Autodesk Fusion 360 part; units mm, degrees
sketch "Sketch1" plane through (0, 0, 0) normal (0, 0, 1) x (1, 0, 0)
  line L0 (-25, 35) -> (19, 35)
  line L1 (19, 35) -> (19, -79)
  line L2 (19, -79) -> (-25, -79)
  line L3 (-25, -79) -> (-25, 35)
  line L4 (-25, 35) -> (-32.5, 35)
  line L5 (-32.5, 35) -> (-32.5, 42.5)
  line L6 (-32.5, 42.5) -> (-25, 42.5)
  line L7 (-25, 42.5) -> (-25, 35)
  line L8 (-32.5, 42.5) -> (26.5, 42.5)
  line L9 (26.5, 42.5) -> (26.5, -86.5)
  line L10 (26.5, -86.5) -> (-32.5, -86.5)
  line L11 (-32.5, -86.5) -> (-32.5, 42.5)
  dimension "d1" = 44
  dimension "d2" = 114
  dimension "d3" = 7.5
  dimension "d4" = 7.5
  dimension "d5" = 59
  dimension "d6" = 129
extrude "Extrude1" add sketch "Sketch1" along normal blind 7 contours L0 L1 L2 L3 | L4 L7 L8 L9 L10 L11 | L4 L5 L6 L7 L8 L11 makes body 1
sketch "Sketch2" plane through (0, 0, 0) normal (0, 0, 1) x (1, 0, 0)
  circle A0 centre (-25, -79) radius 7
  circle A1 centre (19, -79) radius 7
  circle A2 centre (19, 35) radius 7
  circle A3 centre (-25, 35) radius 7
  point P0 (-25, -79)
  point P1 (19, -79)
  point P2 (19, 35)
  point P3 (-25, 35)
  dimension "d9" = 14
  dimension "d10" = 14
  dimension "d11" = 14
  dimension "d12" = 14
extrude "Extrude2" cut sketch "Sketch2" along normal blind 4 contours A0 bodies 1
extrude "Extrude3" cut sketch "Sketch2" along normal blind 4 contours A1 bodies 1
extrude "Extrude4" cut sketch "Sketch2" along normal blind 4 contours A3 bodies 1
extrude "Extrude5" cut sketch "Sketch2" along normal blind 4 contours A2 bodies 1
sketch "Sketch3" plane through (0, 0, 0) normal (0, 0, 1) x (1, 0, 0)
hole "Hole1" at (-25, -79, 4) direction (0, 0, 1) diameter 4 depth 10 tip angle 118 bodies 1
hole "Hole2" at (19, -79, 4) direction (0, 0, 1) diameter 4 depth 10 tip angle 118 bodies 1
hole "Hole3" at (19, 35, 4) direction (0, 0, 1) diameter 4 depth 10 tip angle 118 bodies 1
hole "Hole4" at (-25, 35, 4) direction (0, 0, 1) diameter 4 depth 10 tip angle 118 bodies 1
extrude "Extrude6" add 1 faces at (-12.8333, 42.5, 2.3333) along direction (0, 1, 0) blind 10.5 on bodies 1 bodies 1
extrude "Extrude7" add 1 faces at (6.8333, -86.5, 2.3333) along direction (0, -1, 0) blind 10.5 on bodies 1 bodies 1
sketch "Sketch4" plane through (0, 0, 0) normal (0, 0, -1) x (1, 0, 0)
  circle A0 centre (19, -35) radius 7
  circle A1 centre (-25, -35) radius 7
  circle A2 centre (19, 79) radius 7
  circle A3 centre (-25, 79) radius 7
  line L0 (-32.5, 97) -> (-32.5, -53)
  line L1 (-32.5, -53) -> (26.5, -53)
  line L2 (26.5, -53) -> (26.5, 97)
  line L3 (26.5, 97) -> (-32.5, 97)
  line L4 (-32.5, -53) -> (26.5, -53)
  line L5 (26.5, -53) -> (26.5, 17)
  line L6 (26.5, 17) -> (-32.5, 17)
  line L7 (-32.5, 17) -> (-32.5, -53)
  line L8 (-32.5, 17) -> (-3, 17)
  line L9 (26.5, 17) -> (-3, 17)
  dimension "d37" = 70
hole "Hole5" at (-3, -17, 0) direction (0, 0, 1) diameter 7 depth 10 tip angle 118 bodies 1
sketch "Sketch5" plane through (0, 0, 0) normal (0, 0, -1) x (1, 0, 0)
  line L0 (26.5, 17) -> (-32.5, 17)
  line L1 (-32.5, 17) -> (-32.5, -23)
  line L2 (-32.5, -23) -> (26.5, -23)
  line L3 (26.5, -23) -> (26.5, 17)
  point P0 (26.5, 17)
  dimension "d41" = 59
  dimension "d42" = 40
sketch "Sketch6" plane through (0, 0, 7) normal (0, 0, 1) x (-1, 0, 0)
  circle A0 centre (3, 17) radius 3.5
  circle A1 centre (25, -35) radius 2
  circle A2 centre (-19, -35) radius 2
  circle A3 centre (-19, 79) radius 2
  circle A4 centre (25, 79) radius 2
  line L0 (-26.5, 97) -> (-26.5, -53)
  line L1 (-26.5, -53) -> (32.5, -53)
  line L2 (32.5, -53) -> (32.5, 97)
  line L3 (32.5, 97) -> (-26.5, 97)
  line L4 (-26.5, 17) -> (32.5, 17)
  line L5 (32.5, 17) -> (32.5, 57)
  line L6 (32.5, 57) -> (-26.5, 57)
  line L7 (-26.5, 57) -> (-26.5, 17)
  line L8 (32.5, 57) -> (-26.5, 57)
  line L9 (-26.5, 57) -> (-26.5, 64)
  line L10 (-26.5, 64) -> (32.5, 64)
  line L11 (32.5, 64) -> (32.5, 57)
  point P0 (-26.5, 17)
  dimension "d43" = 40
  dimension "d44" = 7
sketch "Sketch7" plane through (-32.5, 0, 0) normal (-1, 0, 0) x (0, -1, 0)
  line L0 (-53, 0) -> (97, 0)
  line L1 (97, 0) -> (97, 7)
  line L2 (97, 7) -> (-53, 7)
  line L3 (-53, 7) -> (-53, 0)
  line L4 (57, 7) -> (64, 7)
  line L5 (64, 7) -> (64, 0)
  line L6 (64, 0) -> (57, 0)
  line L7 (57, 0) -> (57, 7)
  point P0 (57, 7)
sketch "Sketch8" plane through (26.5, 0, 0) normal (1, 0, 0) x (0, 1, 0)
  line L0 (-97, 0) -> (53, 0)
  line L1 (53, 0) -> (53, 7)
  line L2 (53, 7) -> (-97, 7)
  line L3 (-97, 7) -> (-97, 0)
  line L4 (-64, 7) -> (-57, 7)
  line L5 (-57, 7) -> (-57, 0)
  line L6 (-57, 0) -> (-64, 0)
  line L7 (-64, 0) -> (-64, 7)
  point P0 (-64, 7)
  point P1 (-57, 0)
extrude "Extrude8" add sketch "Sketch8" along normal blind 7 separate body contours L0 L2 L4 L5 L6 L7 | L0 L1 L2 L5 makes body 2
sketch "Sketch9" plane through (0, 0, 0) normal (0, 0, -1) x (1, 0, 0)
  line L0 (-32.5, 57) -> (26.5, 57)
  line L1 (26.5, 57) -> (26.5, 64)
  line L2 (26.5, 64) -> (-32.5, 64)
  line L3 (-32.5, 64) -> (-32.5, 57)
  point P0 (-32.5, 57)
  point P1 (26.5, 64)
extrude "Extrude9" add sketch "Sketch7" along normal blind 7 separate body contours L0 L2 L3 L7 | L0 L2 L4 L5 L6 L7 makes body 3
sketch "Sketch10" plane through (0, 0, 0) normal (0, 0, -1) x (1, 0, 0)
  line L0 (26.5, 64) -> (26.5, -53)
  line L1 (26.5, -53) -> (33.5, -53)
  line L2 (33.5, -53) -> (33.5, 64)
  line L3 (33.5, 64) -> (26.5, 64)
  line L4 (-32.5, -53) -> (-39.5, -53)
  line L5 (-39.5, -53) -> (-39.5, -23)
  line L6 (-39.5, -23) -> (-32.5, -23)
  line L7 (-32.5, -23) -> (-32.5, -53)
  line L8 (33.5, -53) -> (26.5, -53)
  line L9 (26.5, -53) -> (26.5, -23)
  line L10 (26.5, -23) -> (33.5, -23)
  line L11 (33.5, -23) -> (33.5, -53)
  line L12 (-32.5, -23) -> (-39.5, -23)
  line L13 (-39.5, -23) -> (-39.5, 64)
  line L14 (-39.5, 64) -> (-32.5, 64)
  line L15 (-32.5, 64) -> (-32.5, -23)
  line L16 (33.5, -23) -> (26.5, -23)
  line L17 (26.5, -23) -> (26.5, 64)
  line L18 (26.5, 64) -> (33.5, 64)
  line L19 (33.5, 64) -> (33.5, -23)
  point P0 (-32.5, -53)
  point P1 (26.5, -23)
  point P2 (-39.5, 64)
  dimension "d49" = 30
extrude "Extrude10" add sketch "Sketch9" sketch "Sketch10" along normal blind 15 of sketch 2 contours L0 L2 L3 L10 L16 L17 L18 L19 | L6 L12 L13 L14 L15 bodies 1 2 3
extrude "Extrude11" add sketch "Sketch8" along normal blind 7 contours L0 L2 L3 L7 bodies 1
extrude "Extrude12" add sketch "Sketch7" along normal blind 7 contours L0 L1 L2 L5 bodies 1
extrude "Extrude13" add 1 faces at (-3, -58.4478, 7) along direction (0, 0, 1) blind 2 on bodies 1 bodies 1
sketch "Sketch11" plane through (0, 0, -15) normal (0, 0, -1) x (1, 0, 0)
  line L0 (-32.5, 57) -> (26.5, 57)
  line L1 (26.5, 57) -> (26.5, -23)
  line L2 (26.5, -23) -> (33.5, -23)
  line L3 (33.5, -23) -> (33.5, 64)
  line L4 (33.5, 64) -> (-39.5, 64)
  line L5 (-39.5, 64) -> (-39.5, -23)
  line L6 (-39.5, -23) -> (-32.5, -23)
  line L7 (-32.5, -23) -> (-32.5, 57)
  line L8 (-32.5, 57) -> (-39.5, 57)
  line L9 (-39.5, 57) -> (-39.5, 64)
  line L10 (-39.5, 64) -> (-32.5, 64)
  line L11 (-32.5, 64) -> (-32.5, 57)
  line L12 (26.5, 57) -> (33.5, 57)
  line L13 (33.5, 57) -> (33.5, 64)
  line L14 (33.5, 64) -> (26.5, 64)
  line L15 (26.5, 64) -> (26.5, 57)
  line L16 (26.5, 57) -> (-32.5, 57)
  line L17 (-32.5, 57) -> (-32.5, 64)
  line L18 (-32.5, 64) -> (26.5, 64)
  line L19 (26.5, 64) -> (26.5, 57)
  line L20 (33.5, 57) -> (-39.5, 57)
  line L21 (-39.5, 57) -> (-39.5, 49)
  line L22 (-39.5, 49) -> (33.5, 49)
  line L23 (33.5, 49) -> (33.5, 57)
  dimension "d58" = 8
extrude "Extrude14" add sketch "Sketch11" along normal blind 7 separate body contours L0 L4 L11 L15 L16 L17 L18 L19 L20 | L4 L5 L8 L9 L10 L11 L17 L20 | L3 L4 L12 L13 L14 L15 L19 L20 makes body 4
extrude "Extrude15" add 1 faces at (9.1667, -57, -17.3333) along direction (0, 1, 0) blind 8 on bodies 4 bodies 1 4
Model file for the job. Use its own axes, mm. A direction names the side the tool comes from. Give positions to 0.01 mm unless a question says otherwise; leave off trailing zeros. Order: outer loops, then holes, each group sorted by start corner. A loop starts at its lowest first (then second) coordinate and runs counter-clockwise, first axis right, second up.
1) Wall check: probe 1 along Y at (x, z) = (19, 1.85); probe 2 along Y at (x, z) = (-25, 7.65); probe 3 along X at (y, z) = (35, 7.55). Give the ranges that are in metal, low to high.
2) Saw through at D-D, the plane z = -4.5. Write the cut outline in (x, y), then the cut area to 3 significant figures.
3) Mould opens along Y. For faces 1 (the flat face through (-3, -57, -7)), 2 (the cylindrical face through (13.84, 30.27, 1.97)), 3 (the flat face through (30, -14, -15)), 4 (the cylindrical face through (-25.91, -85.94, 1.97)) say: +Y half, -Y half, draft (parallel to the pull), parting line (faces both ways), or undercut.
4) 3-axis set-ups, long thin cutter, end or side, ignore diameter. For faces 5 (the flat face through (-24, -77, 4)), 6 (the flat face through (-36, -14, -15)), 7 (the flat face through (-2, -80, 0)), 8 (the flat face through (-4, -97, 4)), 9 (the flat face through (-39.5, -23, -3)): which of +Z, -Z, +X, -X, +Y, -Y reach the whole face in a straight line?
5) Saw through at A-A, the plane y = -17. Write the cut outline in (x, z), then the cut area to 3 significant figures.
6) Saw through at C-C, the plane x = 19. Write the cut outline in (y, z), then the cut area to 3 significant figures.
7) Pin check, flat tips, straight feed: pin 1 (15.5 mm diameter, centred on x = 18.5, y = -82, fed in from -Z); pin 2 (12 mm diameter, centred on x = -31, y = 12, fed in from -Z); pin 3 (4 mm diameter, centred on x = 20, z = -12.5, fed in from -Y). Stop position of each tip, or through.
8) Saw through at B-B, the plane x = -3. Write the cut outline in (y, z).
Computed:
1. probe 1: y = -97 to -86, -72 to 28, 42 to 53
1. probe 2: y = -97 to -81, -77 to 33, 37 to 53
1. probe 3: x = -39.5 to -27, -23 to 17, 21 to 33.5
2. outline: (-39.5, -64) - (33.5, -64) - (33.5, 23) - (26.5, 23) - (26.5, -57) - (-32.5, -57) - (-32.5, 23) - (-39.5, 23) - close
2. area: 1,630 mm2
3. face 1: +Y half
3. face 2: undercut
3. face 3: draft
3. face 4: undercut
4. face 5: -Z
4. face 6: -Z, +X, -X, +Y
4. face 7: -Z, +X, -X, -Y
4. face 8: +Z, -Z, +X, -X, -Y
4. face 9: +Z, -Z, -X, +Y, -Y
5. outline: (-39.5, -15) - (-32.5, -15) - (-32.5, 0) - (-6.5, 0) - (-6.5, 9) - (-39.5, 9) - close; (0.5, 0) - (26.5, 0) - (26.5, -15) - (33.5, -15) - (33.5, 9) - (0.5, 9) - close
5. area: 804 mm2
6. outline: (-97, 0) - (-86, 0) - (-86, 4) - (-81, 4) - (-81, 9) - (-97, 9) - close; (-77, 4) - (-72, 4) - (-72, 0) - (-64, 0) - (-64, -22) - (-49, -22) - (-49, -15) - (-57, -15) - (-57, 0) - (28, 0) - (28, 4) - (33, 4) - (33, 9) - (-77, 9) - close; (37, 4) - (42, 4) - (42, 0) - (53, 0) - (53, 9) - (37, 9) - close
6. area: 1,410 mm2
7. pin 1: stops at z = 0
7. pin 2: stops at z = -15
7. pin 3: stops at y = -64
8. outline: (-97, 0) - (-64, 0) - (-64, -22) - (-49, -22) - (-49, -15) - (-57, -15) - (-57, 0) - (-20.5, 0) - (-20.5, 9) - (-97, 9) - close; (-13.5, 0) - (53, 0) - (53, 9) - (-13.5, 9) - close
